Input: part model. Units: mm. Frame: model coordinates. A direction names the side the tool comes from. Give positions to 0.01 mm unless a question says otherwise; leave off trailing zeros. Loops run counter-clockwise (first coordinate to the right, second up) from the corner with the lowest first, then second, coordinate; pieces in that order, holes last. Notation, with made-up numbers: (15, 80.25) - (63, 80.25) arc R32 ccw to (63, 114.25) - close; hole circle Ø4 at (-0.75, 20). An arc over 180 degrees is marked (long way). Answer as a JSON object with one key per item and string values. Group by question number.
(1) Material intervals for L1, parallel to Y at x = 4.75, z = 0; L2, parallel to X at y = -6, z = 5.25; L3, parallel to Z at x = 12.5, y = -1.5, sorted ascending.
(2) Pin query (flat end, axial travel): P1, Ø3, axis at x = 8.5, z = 1.5, coming from the -Y side; P2, Ø1, axis at x = 6, y = 0.5, coming from the -Z side; P3, Ø6, axis at x = 8.5, y = -1.5, coming from the +Z side. Return the tip coordinate at first contact, or that it passes through.
(3) Access query for faces 5 (the cylindrical face through (6.93, -1.802, 5.723)), 6 (the cylindrical face through (7, 0, -5)). Directions: +Z, -Z, +X, -X, +Y, -Y. A direction counts if a zero-diameter tool reaches every point of the face in a straight line with its end or side. Return the directions, or none.
(4) Mould query, pull axis X, two halves, no side actions, for faces 1 (the flat face through (14, 5.2, 0.1)), 2 (the flat face through (13, 6, 4)), 3 (the cylindrical face through (13.49, 7.81, -1.73)), 4 (the flat face through (0, 5.2, -0.1)). Classes: +X half, -X half, draft (parallel to the pull), parting line (faces both ways), or undercut.
(5) Section query C-C (x = 3.75). Return loops of the section in (y, z).
(6) Section query A-A (z = 0). Return loops of the section in (x, y), plus the area to 3 significant figures.
(7) Section query D-D (x = 1.5). Return loops of the section in (y, z).
```python
from build123d import *

# Parameters (mm, degrees)
FILLET1_R = 1


with BuildPart() as part:
    # Sketch1 → Revolve1 (revolve)
    with BuildSketch(Plane(origin=(0, 0, 0), x_dir=(1, 0, 0), z_dir=(0, 1, 0)), mode=Mode.PRIVATE) as revolve1_sk:
        Polygon((0, 8), (0, 5), (14, 5), (14, 8), (13, 8), (13, 6), (1, 6), (1, 8), align=None)
    revolve(revolve1_sk.sketch.rotate(Axis((0, 0, 0), (1, 0, 0)), 180), axis=Axis((0, 0, 0), (1, 0, 0)))

    # Fillet1
    fillet1_edges = [part.edges().sort_by_distance(p)[0] for p in [
        (1, 0, -6),
        (13, 0, -6),
    ]]
    fillet(fillet1_edges, radius=FILLET1_R)


solid = part.part
```
Recorded:
{
 "1": {"L1": "y = -6 to -5, 5 to 6", "L2": "x = 0 to 1, 13 to 14", "L3": "z = -5.95 to -4.77, 4.77 to 5.95"},
 "2": {"P1": "stops at y = -6", "P2": "stops at z = -6", "P3": "stops at z = 6"},
 "3": {"face 5": "none", "face 6": "+X, -X"},
 "4": {"face 1": "+X half", "face 2": "undercut", "face 3": "draft", "face 4": "-X half"},
 "5": {"outline": "circle Ø12 at (0, 0); hole circle Ø10 at (0, 0)"},
 "6": {"outline": "(0, -8) - (1, -8) - (1, -7) arc R1 cw to (2, -6) - (12, -6) arc R1 cw to (13, -7) - (13, -8) - (14, -8) - (14, -5) - (0, -5) - close; (0, 5) - (14, 5) - (14, 8) - (13, 8) - (13, 7) arc R1 cw to (12, 6) - (2, 6) arc R1 cw to (1, 7) - (1, 8) - (0, 8) - close", "area": "36.9 mm^2"},
 "7": {"outline": "circle Ø12.27 at (0, 0); hole circle Ø10 at (0, 0)"}
}
